Print and shaded views of the part. All mm, measured from the part's lowest x, y and z. A direction names the side the tool comes from. Round coordinates to 2 decimals unless told otherwise and drop trailing zeros. Order: outer loops, then holes, each group sorted by start corner. A loop starts at its lowest first (then second) coordinate and runs counter-clockwise, first axis right, second up. Notation, with made-up numbers: M 38,56.25 L 72,56.25 A34 ccw 72,90.25 Z; hole C 59,2.25 d3. An arc over 180 degrees is marked long. Write each question's results on one line, items separated by ' | '. Start each with the question number.
1. Probe L1, parallel to X at y = 8, z = 10; L2, parallel to Z at x = 190, y = 4.75; L3, parallel to X at y = 1, z = 54. List the from-to ranges inside material, lowest first. Write a range as [from, to].
2. Band-saw the part on A-A, the plane z = 10. List the corners of the cut face in (x, y).
3. Drop flat-ended pins along their axis: pin 1 Ø3 at (x, z) = (92, 83.5) entering from +Y; pin 2 Ø9 at (x, z) = (135, 108.5) entering from -Y; pin 3 Ø4.5 at (x, z) = (190, 10) entering from +Y; pin 4 Ø1.6 at (y, z) = (0.5, 109) entering from +X. Give the stop position or say it passes through.
4. Band-saw the part on C-C, the plane z = 127. List the corners of the cut face in (x, y), then the cut area to 3 significant figures.
5. Which spindle directions (+Z, -Z, +X, -X, +Y, -Y) get a long thin tool onto all of the face, cutting with end or side? Do the marked faces 4, 5, 6, 7 and 8. Say none if no direction does.
6. Band-saw the part on D-D, the plane x = 133.5. List the corners of the cut face in (y, z), then the cut area to 3 significant figures.
7. Band-saw the part on B-B, the plane x = 190. List the corners of the cut face in (y, z), then the cut area to 3 significant figures.
8. Two-plate mould, pull along X, no slides. Class the marked faces 1, 2 and 3: +X half, -X half, draft (parallel to the pull), parting line (faces both ways), or undercut.
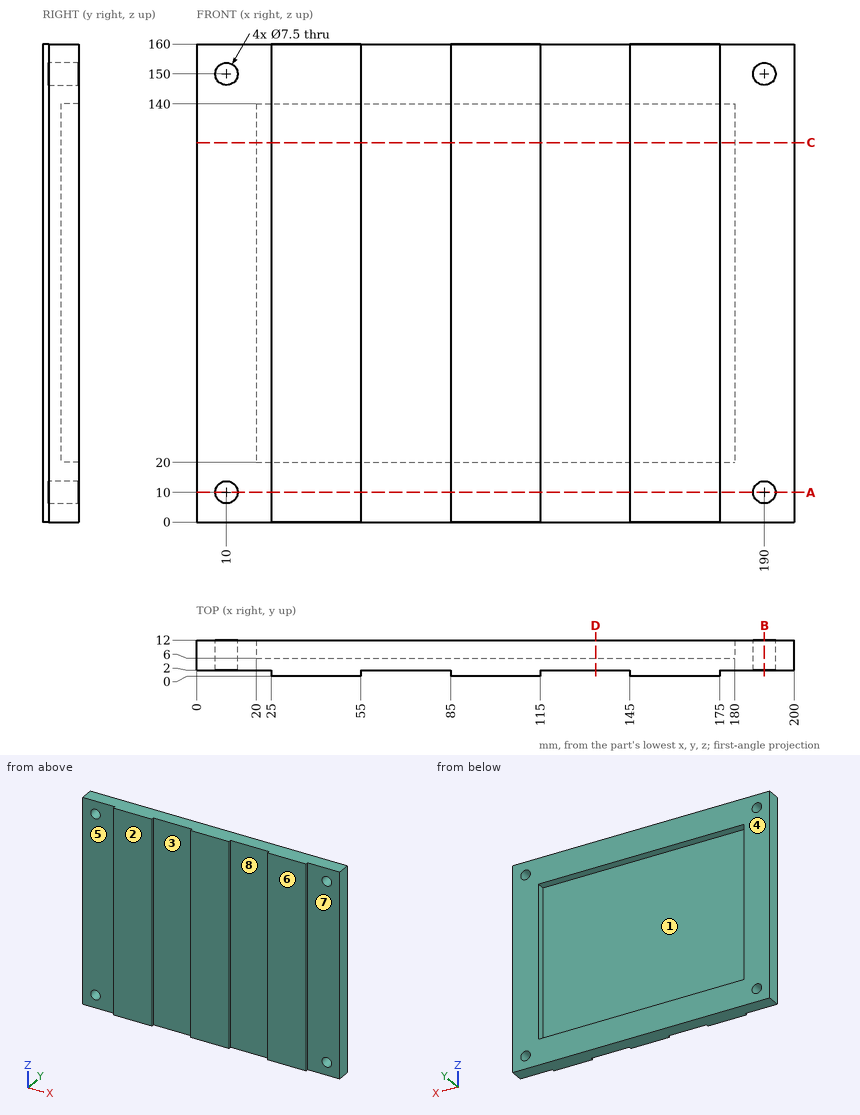
Solution:
1) L1: [0, 6.25], [13.75, 186.25], [193.75, 200] | L2: [0, 6.25], [13.75, 146.25], [153.75, 160] | L3: [25, 55], [85, 115], [145, 175]
2) outline: M 0,2 L 6.25,2 L 6.25,12 L 0,12 Z; M 13.75,2 L 25,2 L 25,0 L 55,0 L 55,2 L 85,2 L 85,0 L 115,0 L 115,2 L 145,2 L 145,0 L 175,0 L 175,2 L 186.25,2 L 186.25,12 L 13.75,12 Z; M 193.75,2 L 200,2 L 200,12 L 193.75,12 Z
3) pin 1: y = 6 | pin 2: y = 2 | pin 3: through | pin 4: x = 175
4) outline: M 0,2 L 25,2 L 25,0 L 55,0 L 55,2 L 85,2 L 85,0 L 115,0 L 115,2 L 145,2 L 145,0 L 175,0 L 175,2 L 200,2 L 200,12 L 180,12 L 180,6 L 20,6 L 20,12 L 0,12 Z | area: 1,220 mm^2
5) face 4: +Z, -Z, +X, -X, +Y | face 5: +Z, -Z, -X, -Y | face 6: +Z, -Z, +X, -X, -Y | face 7: +Z, -Z, +X, -Y | face 8: +Z, -Z, -Y
6) outline: M 2,0 L 12,0 L 12,20 L 6,20 L 6,140 L 12,140 L 12,160 L 2,160 Z | area: 880 mm^2
7) outline: M 2,0 L 12,0 L 12,6.25 L 2,6.25 Z; M 2,13.75 L 12,13.75 L 12,146.25 L 2,146.25 Z; M 2,153.75 L 12,153.75 L 12,160 L 2,160 Z | area: 1,450 mm^2
8) face 1: undercut | face 2: draft | face 3: undercut
